Work out the finished part from the listing and answer in its coordinate system (mm). Face numbers are marked on the shaded views. A direction names the side the tool comes from. Round coordinates to 2 decimals unless told otherwise and drop trailing zeros. Write each loop counter-clockwise with the first axis right and the second up, starting at its lowest first coordinate (ties: lowest second). Pieces come first, ordered by that corner, then holes.
1. Find section D-D (y = 4). Write down the section's boundary in (x, z), and give its area (3 significant figures).
2. Straight lines are drawn through the part: probe 1 along X at (y, z) = (12, 0); probe 2 along X at (y, z) = (33, 0). For each, find the intervals that lie inside material, in ascending order.
3. Determine the mould class of the marked faces 3 and 4 for opening direction Z: pulls with the +Z half, pulls with the -Z half, needs draft (parallel to the pull), parting line crosses it, or undercut.
4. A tool of negligible diameter and unlimited length cuts with its end or side. For the marked faces 1 and 2, from which of +Z, -Z, +X, -X, +Y, -Y can it reach the whole face along a straight path? Write none if from no direction.
5. Find section C-C (y = 29). Write down the section's boundary in (x, z), and give its area (3 significant figures).
6. Flat-ended cylindrical pins translate along their axes: pin 1 Ø4 at (x, z) = (6.5, -26) entering from -Y; pin 2 Ø1.5 at (x, y) = (-11.5, 27) entering from +Z; pin 3 Ø4 at (x, y) = (-16.5, 7) entering from +Z. Find the tip coordinate at first contact, or state that the pin passes through.
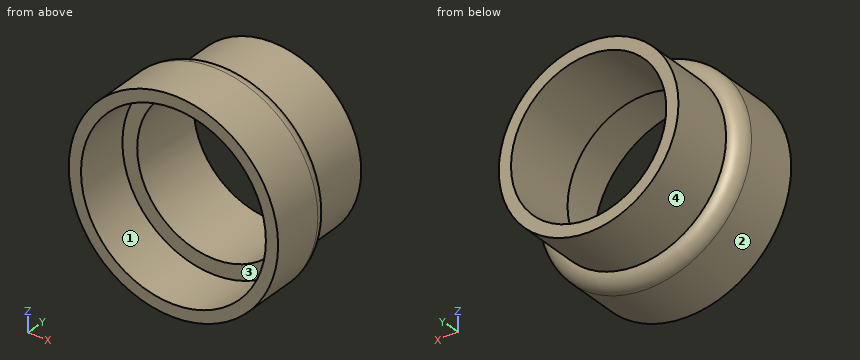
Autodesk Inventor part; units mm, degrees
ref_plane "YZ Plane" through (0, 0, 0) normal (1, 0, 0) x (0, 1, 0)
ref_plane "XZ Plane" through (0, 0, 0) normal (0, 1, 0) x (-1, 0, 0)
ref_plane "XY Plane" through (0, 0, 0) normal (0, 0, 1) x (1, 0, 0)
sketch "Sketch1" plane through (0, 0, 0) normal (0, 0, 1) x (1, 0, 0)
  line L0 (0, 0) -> (0, 29.5332)
  line L1 (29.4, 44) -> (29.4, 22.6)
  line L2 (29.4, 22.6) -> (29.4875, 22.6)
  line L3 (34.25, 17.8375) -> (34.25, 0)
  line L4 (34.25, 0) -> (30.25, 0)
  line L5 (25.4, 44) -> (29.4, 44)
  line L6 (25.4, 44) -> (25.4, 18.6)
  line L7 (25.4, 18.6) -> (30.25, 18.6)
  line L8 (30.25, 18.6) -> (30.25, 0)
  arc A0 (34.25, 17.8375) -> (29.4875, 22.6) centre (29.4875, 17.8375) ccw
  dimension "d0" = 25.4
  dimension "d1" = 30.25
  dimension "d2" = 4
  dimension "d3" = 4
  dimension "d4" = 25.4
  dimension "d5" = 44
  dimension "d6" = 0
  dimension "d7" = 4
  dimension "d8" = 4.7625
revolve "Revolution1" add sketch "Sketch1" angle 360 about axis through (0, 0, 0) along (0, 1, 0)
properties part number "Male Adaptor to Water Sensor"
Worked answers:
1. outline: circle Ø68.5 at (0, 0); hole circle Ø60.5 at (0, 0)
1. area: 811 mm2
2. probe 1: x = -34.25 to -30.25, 30.25 to 34.25
2. probe 2: x = -29.4 to -25.4, 25.4 to 29.4
3. face 3: undercut
3. face 4: parting line crosses it
4. face 1: -Y
4. face 2: +Y, -Y
5. outline: circle Ø58.8 at (0, 0); hole circle Ø50.8 at (0, 0)
5. area: 689 mm2
6. pin 1: stops at y = 18.6
6. pin 2: stops at z = 27.36
6. pin 3: stops at z = 31.03
